Input: dimensioned drawing with shaded views. Units: mm. Origin: part minimum x, y, z. A direction names the side the tool comes from. Round coordinates to 2 decimals unless told otherwise and drop trailing zeros. Order: outer loops, then holes, each group sorted by start corner. A loop starts at its lowest first (then second) coordinate and runs counter-clockwise, first axis right, second up. Notation, with made-up numbers: (41.5, -26.75) - (86.5, -26.75) arc R21 cw to (86.5, -22.75) - close; hole circle Ø2 at (50.25, 83). An arc over 180 degrees is marked (long way). Put each result on its own line as item: value. Start each with the question number.
(1) Section A-A (x = 3). Output: boundary loops of the cut face in (y, z), and give its area (3 significant figures).
(2) Section C-C (y = 20.5). Output: boundary loops of the cut face in (x, z).
(3) Section D-D (y = 3). Output: boundary loops of the cut face in (x, z), and give its area (3 significant figures).
(4) Section B-B (z = 4). Output: boundary loops of the cut face in (x, y).
(5) Material intervals for L1, parallel to X at y = 35, z = 1.5; L2, parallel to Y at x = 35, z = 1.25; L3, parallel to Y at x = 22.5, z = 3.25, sorted ascending. Write a range as [from, to].
(6) Pull-direction query (Y, two-part tool) for the marked faces 3, 4, 5 and 6; classes: released by +Y, released by -Y, zero draft, split by the parting line, or undercut.
(7) Access query for the marked faces 1 and 2. Directions: +Z, -Z, +X, -X, +Y, -Y. A direction counts if a zero-diameter tool reaches every point of the face in a straight line with its end or side. Return the directions, or none.
(8) Pin query (flat end, axial travel): P1, Ø1.8, axis at x = 4, y = 36.5, coming from the +Z side; P2, Ø5, axis at x = 33.5, y = 36, coming from the +Z side; P3, Ø1, axis at y = 10.5, z = 4.5, coming from the +X side. Return the tip coordinate at first contact, or that it passes through.
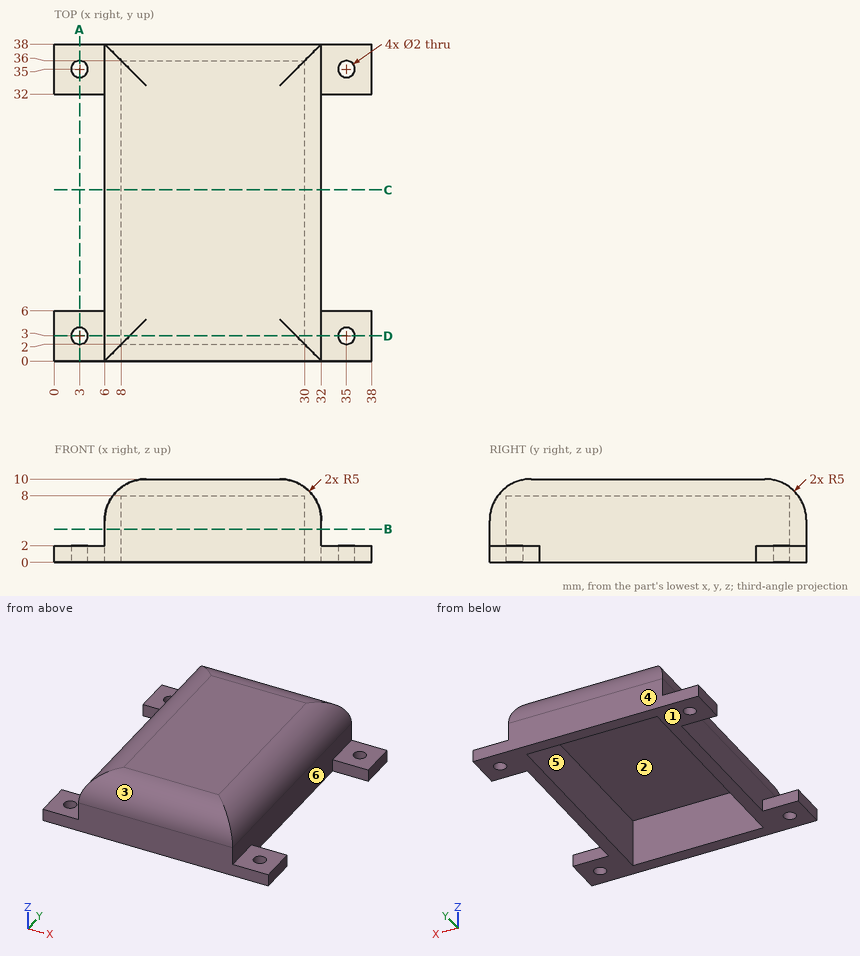
Checks:
1. outline: (0, 0) - (2, 0) - (2, 2) - (0, 2) - close; (4, 0) - (6, 0) - (6, 2) - (4, 2) - close; (32, 0) - (34, 0) - (34, 2) - (32, 2) - close; (36, 0) - (38, 0) - (38, 2) - (36, 2) - close
1. area: 16.0 mm²
2. outline: (6, 0) - (8, 0) - (8, 8) - (30, 8) - (30, 0) - (32, 0) - (32, 5) arc R5 ccw to (27, 10) - (11, 10) arc R5 ccw to (6, 5) - close
3. outline: (0, 0) - (2, 0) - (2, 2) - (0, 2) - close; (4, 0) - (8, 0) - (8, 8) - (30, 8) - (30, 0) - (34, 0) - (34, 2) - (32, 2) - (32, 5) arc R5 ccw to (29, 9.58) - (9, 9.58) arc R5 ccw to (6, 5) - (6, 2) - (4, 2) - close; (36, 0) - (38, 0) - (38, 2) - (36, 2) - close
3. area: 81.5 mm²
4. outline: (6, 0) - (32, 0) - (32, 38) - (6, 38) - close; hole (8, 2) - (30, 2) - (30, 36) - (8, 36) - close
5. L1: x = [0, 2], [4, 8], [30, 34], [36, 38]
5. L2: y = [0, 2], [4, 6], [32, 34], [36, 38]
5. L3: y = [0, 2], [36, 38]
6. face 3: released by -Y
6. face 4: released by +Y
6. face 5: undercut
6. face 6: undercut
7. face 1: -Z, +X, -X, +Y, -Y
7. face 2: -Z
8. P1: stops at z = 2
8. P2: stops at z = 8
8. P3: stops at x = 32
